Can you work these out from the model? Positions are in its coordinate system, mm. A direction names the side the tool comes from. Give positions to 0.01 mm unless a question says otherwise; leave off trailing zeros. Order: outer loops, then holes, each group sorted by start corner. A loop starts at its lowest first (then second) coordinate and runs counter-clockwise, first axis right, second up.
Item 1: I'm going to push flat-ended pins straight in: pin 1 Ø8 at (x, z) = (-5.5, -2) entering from -Y; pin 2 Ø4.5 at (x, z) = (0, 0) entering from +Y. Where does each tip first touch, or does it pass through?
Item 2: I want a section at A-A, the plane x = 29.5. Write out the boundary of the cut face in (y, z).
Item 3: If we mould it in two halves opening along Z, with no side actions, what happens to faces 5 (the flat face through (0, 53, 9)), 6 (the flat face through (0, 53, -9)), 7 (the cylindrical face through (48.683, -44.925, 0.182))? For each: +Z half, -Z half, draft (parallel to the pull), parting line (faces both ways), or undercut.
Item 4: If I drill on line 1 along X through (y, z) = (-26.75, 0); line 2 along Y through (x, z) = (30, 0); line 3 along X through (y, z) = (-48, -6.5), over which ranges is the centre line in solid material (lowest first)?
Item 5: Which directions (+Z, -Z, +X, -X, +Y, -Y) give clear straight access to the entire face, cutting with the end or side of a thin tool? Please do faces 1 (the flat face through (-30, -47.5, 0)), 2 (the cylindrical face through (45.18, -1.08, -4.88)), 3 (the cylindrical face through (-52.57, 19.905, 1.468)), 4 (the flat face through (7.5, -46, 0)).
Item 6: I want a section at C-C, the plane x = -27.5. Write out the boundary of the cut face in (y, z).
Item 7: I want a section at B-B, the plane y = 23.6. Write out the boundary of the cut face in (x, z).
```python
from build123d import *

# Parameters (mm, degrees)
SKETCH1_W           = 115
SKETCH1_H           = 115
SKETCH1_W_2         = 95
SKETCH1_H_2         = 95
BOSS_EXTRUDE1_DEPTH = 26
SKETCH10_W          = 40
SKETCH10_H          = 26
BOSS_EXTRUDE4_DEPTH = 27
SKETCH3_W           = 15
SKETCH3_H           = 15
CUT_EXTRUDE1_DEPTH  = 24
FILLET1_R           = 10
CHAMFER1_SIZE       = 10
SKETCH4_R           = 3.15
CUT_EXTRUDE3_DEPTH  = 57.5
SKETCH9_R           = 4
CUT_EXTRUDE7_DEPTH  = 30
FILLET5_R           = 2
SKETCH11_W          = 26
SKETCH11_H          = 20
BOSS_EXTRUDE5_DEPTH = 25
FILLET6_R           = 2
SKETCH13_R          = 5
CUT_EXTRUDE9_DEPTH  = 25
SKETCH14_R          = 2.5
CUT_EXTRUDE10_DEPTH = 15
CUT_EXTRUDE11_DEPTH = 10
SKETCH16_R          = 2.4
CUT_EXTRUDE12_DEPTH = 30


with BuildPart() as part:
    # Sketch1 → Boss-Extrude1 (new body)
    with BuildSketch(Plane.XY.offset(-13)):
        Rectangle(SKETCH1_W, SKETCH1_H)
        Rectangle(SKETCH1_W_2, SKETCH1_H_2, mode=Mode.SUBTRACT)
    extrude(amount=BOSS_EXTRUDE1_DEPTH)

    # Sketch10 → Boss-Extrude4 (add)
    with BuildSketch(Plane(origin=(0, -24.638, 0), x_dir=(1, 0, 0), z_dir=(0, 1, 0))):
        Rectangle(SKETCH10_W, SKETCH10_H)
    extrude(amount=-BOSS_EXTRUDE4_DEPTH)

    # Sketch3 → Cut-Extrude1 (cut)
    with BuildSketch(Plane(origin=(0, -57.5, 0), x_dir=(-1, 0, 0), z_dir=(0, -1, 0))):
        Rectangle(SKETCH3_W, SKETCH3_H)
    extrude(amount=-CUT_EXTRUDE1_DEPTH, mode=Mode.SUBTRACT)

    # Fillet1
    fillet1_edges = [part.edges().sort_by_distance(p)[0] for p in [
        (-57.5, 57.5, 0),
        (57.5, 57.5, 0),
        (57.5, -57.5, 0),
        (-57.5, -57.5, 0),
    ]]
    fillet(fillet1_edges, radius=FILLET1_R)

    # Chamfer1
    chamfer1_edges = [part.edges().sort_by_distance(p)[0] for p in [
        (-47.5, 47.5, 0),
        (-47.5, -47.5, 0),
        (47.5, -47.5, 0),
        (47.5, 47.5, 0),
    ]]
    chamfer(chamfer1_edges, length=CHAMFER1_SIZE)

    # Sketch4 → Cut-Extrude3 (cut, symmetric)
    with BuildSketch(Plane.XY):
        with Locations(Location((-48, 48, 0), (0, 0, 180))):
            Circle(SKETCH4_R)
        with Locations(Location((48, 48, 0), (0, 0, 180))):
            Circle(SKETCH4_R)
        with Locations(Location((48, -48, 0), (0, 0, 180))):
            Circle(SKETCH4_R)
        with Locations(Location((-48, -48, 0), (0, 0, 180))):
            Circle(SKETCH4_R)
    extrude(amount=CUT_EXTRUDE3_DEPTH, both=True, mode=Mode.SUBTRACT)

    # Sketch9 → Cut-Extrude7 (cut)
    with BuildSketch(Plane.ZY.offset(57.5)):
        with Locations(Location((3, 23.6, 0), (0, 0, 270))):
            Circle(SKETCH9_R)
    extrude(amount=-CUT_EXTRUDE7_DEPTH, mode=Mode.SUBTRACT)

    # Fillet5
    fillet5_edges = [part.edges().sort_by_distance(p)[0] for p in [
        (20, -47.5, 0),
        (-20, -47.5, 0),
        (-20, -24.638, 0),
        (20, -24.638, 0),
    ]]
    fillet(fillet5_edges, radius=FILLET5_R)

    # Sketch11 → Boss-Extrude5 (add)
    with BuildSketch(Plane(origin=(25.5, 0, 0), x_dir=(0, 0, -1), z_dir=(1, 0, 0))):
        Rectangle(SKETCH11_W, SKETCH11_H)
    extrude(amount=BOSS_EXTRUDE5_DEPTH)

    # Fillet6
    fillet6_edges = [part.edges().sort_by_distance(p)[0] for p in [
        (25.5, -10, 0),
        (25.5, 10, 0),
    ]]
    fillet(fillet6_edges, radius=FILLET6_R)

    # Sketch13 → Cut-Extrude9 (cut)
    with BuildSketch(Plane(origin=(57.5, 0, 0), x_dir=(0, 0, -1), z_dir=(1, 0, 0))):
        with Locations(Location((0, 0, 0), (0, 0, 90))):
            Circle(SKETCH13_R)
    extrude(amount=-CUT_EXTRUDE9_DEPTH, mode=Mode.SUBTRACT)

    # Sketch14 → Cut-Extrude10 (cut)
    with BuildSketch(Plane(origin=(25.5, 0, 0), x_dir=(0, 0, -1), z_dir=(1, 0, 0))):
        with Locations(Location((0, 0, 0), (0, 0, 180))):
            Circle(SKETCH14_R)
    extrude(amount=CUT_EXTRUDE10_DEPTH, mode=Mode.SUBTRACT)

    # Sketch15 → Cut-Extrude11 (cut)
    with BuildSketch(Plane(origin=(0, 57.5, 0), x_dir=(1, 0, 0), z_dir=(0, 1, 0))):
        with BuildLine():
            Line((-10, 9), (10, 9))
            ThreePointArc((10, 9), (19, 0), (10, -9))
            Line((10, -9), (-10, -9))
            ThreePointArc((-10, -9), (-19, 0), (-10, 9))
        make_face()
    extrude(amount=-CUT_EXTRUDE11_DEPTH, mode=Mode.SUBTRACT)

    # Sketch16 → Cut-Extrude12 (cut)
    with BuildSketch(Plane(origin=(0, -24.638, 0), x_dir=(1, 0, 0), z_dir=(0, 1, 0))):
        with Locations(Location((0, 0, 0), (0, 0, 270))):
            Circle(SKETCH16_R)
    extrude(amount=-CUT_EXTRUDE12_DEPTH, mode=Mode.SUBTRACT)


solid = part.part
```
Results list:
1. pin 1: stops at y = -57.5
1. pin 2: passes through
2. outline: (-57.5, -13) - (-47.5, -13) - (-47.5, 13) - (-57.5, 13) - close; (-10, -13) - (10, -13) - (10, 13) - (-10, 13) - close; (47.5, -13) - (57.5, -13) - (57.5, 13) - (47.5, 13) - close; hole circle Ø5 at (0, 0)
3. face 5: undercut
3. face 6: undercut
3. face 7: draft
4. line 1: x = -57.5 to -47.5, -20 to -2.4, 2.4 to 20, 47.5 to 57.5
4. line 2: y = -57.5 to -47.5, -10 to -2.5, 2.5 to 10, 47.5 to 57.5
4. line 3: x = -57.49 to -51.15, -44.85 to -7.5, 7.5 to 44.85, 51.15 to 57.49
5. face 1: +Z, -Z
5. face 2: +X
5. face 3: -X
5. face 4: -Y
6. outline: (-57.5, -13) - (-47.5, -13) - (-47.5, 13) - (-57.5, 13) - close; (47.5, -13) - (57.5, -13) - (57.5, 13) - (47.5, 13) - close
7. outline: (-57.5, -13) - (-47.5, -13) - (-47.5, -1) - (-57.5, -1) - close; (-57.5, 7) - (-47.5, 7) - (-47.5, 13) - (-57.5, 13) - close; (47.5, -13) - (57.5, -13) - (57.5, 13) - (47.5, 13) - close
